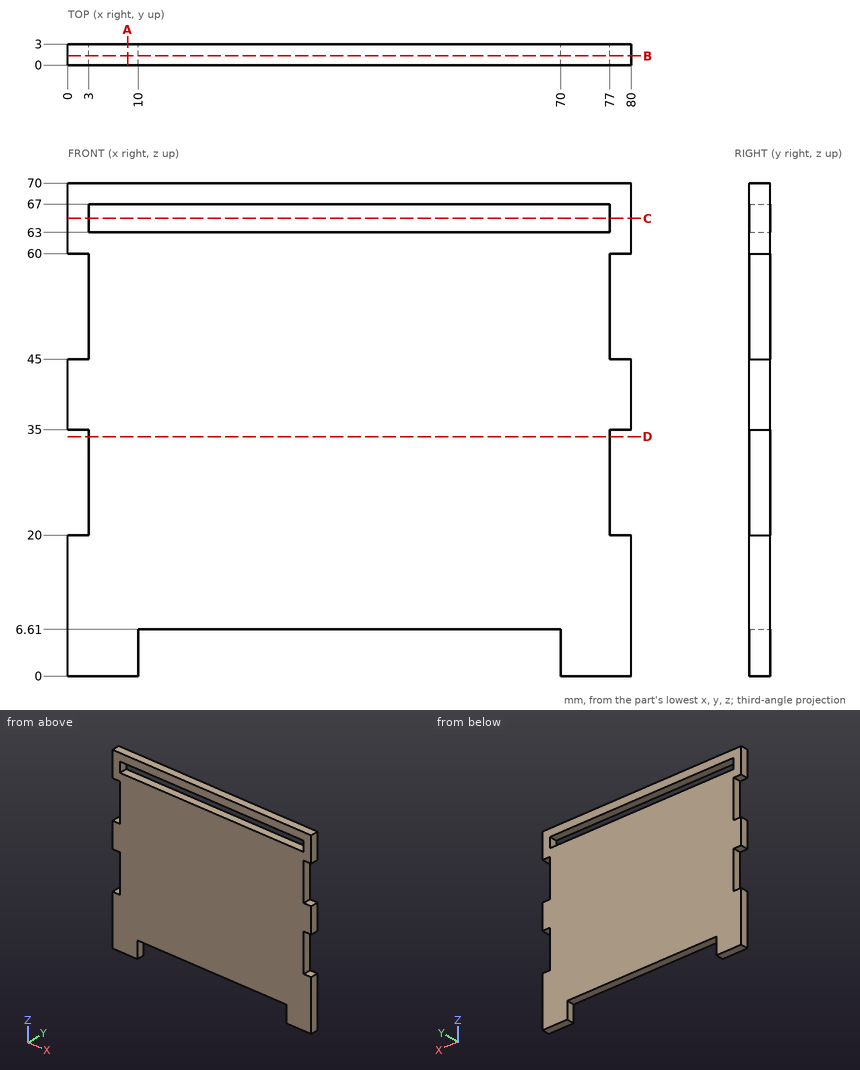
Geometry check sheet. Reference: drawing and pictorial views, mm from the part's lowest x, y, z. Round coordinates to 2 decimals unless told otherwise and drop trailing zeros. Loops run counter-clockwise (first coordinate to the right, second up) from the corner with the lowest first, then second, coordinate; pieces in that order, holes last. Notation, with made-up numbers: (54.5, 15.25) - (71.5, 15.25) arc R21 cw to (71.5, 24.25) - close; hole circle Ø2 at (-8.5, 58.25). An arc over 180 degrees is marked (long way). Answer as CSV lines item,"result".
(1) Cross-section at C-C, the plane z = 65. Enter the section's corners in (x, y), and give its area (3 significant figures).
Output values:
outline,"(0, 0) - (3, 0) - (3, 3) - (0, 3) - close; (77, 0) - (80, 0) - (80, 3) - (77, 3) - close"
area,"18.0 mm²"
(2) Depth check by flat-ended pin: pin 1 Ø1.5 at (y, z) = (1.5, 31) entering from +X; pin 2 Ø1.5 at (x, y) = (19.5, 2) entering from -Z. Enter the tip coordinate at first touch or a pass-through.
Output values:
pin 1,"stops at x = 77"
pin 2,"stops at z = 6.61"
(3) Cross-section at A-A, the plane x = 8.5. Enter the section's corners in (y, z), and give its area (3 significant figures).
Output values:
outline,"(0, 0) - (3, 0) - (3, 63) - (0, 63) - close; (0, 67) - (3, 67) - (3, 70) - (0, 70) - close"
area,"198 mm²"
(4) Material ranges on line 1 along Z through (x, y) = (76, 1); line 2 along Z through (x, y) = (20, 0.6); line 3 along X through (y, z) = (0.55, 46.5), recorded low to high.
Output values:
line 1,"z = 0 to 63, 67 to 70"
line 2,"z = 6.61 to 63, 67 to 70"
line 3,"x = 3 to 77"
(5) Cross-section at D-D, the plane z = 34. Enter the section's corners in (x, y).
Output values:
outline,"(3, 0) - (77, 0) - (77, 3) - (3, 3) - close"
(6) Cross-section at B-B, the plane y = 1.3. Enter the section's corners in (x, z), and give its area (3 significant figures).
Output values:
outline,"(0, 0) - (10, 0) - (10, 6.61) - (70, 6.61) - (70, 0) - (80, 0) - (80, 20) - (77, 20) - (77, 35) - (80, 35) - (80, 45) - (77, 45) - (77, 60) - (80, 60) - (80, 70) - (0, 70) - (0, 60) - (3, 60) - (3, 45) - (0, 45) - (0, 35) - (3, 35) - (3, 20) - (0, 20) - close; hole (3, 63) - (77, 63) - (77, 67) - (3, 67) - close"
area,"4,730 mm²"
